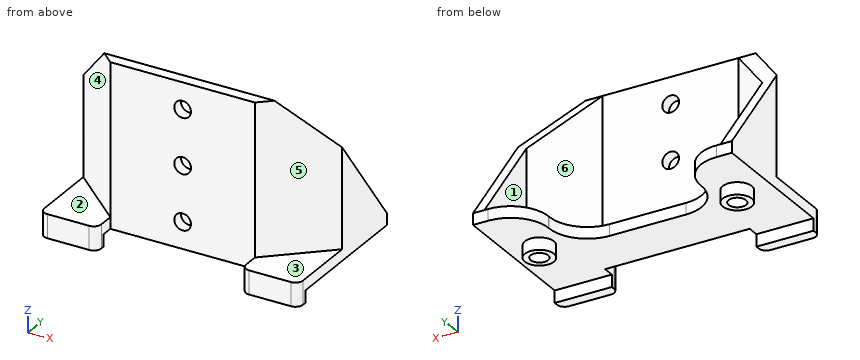
from build123d import *

# Parameters (mm, degrees)
F4_DEPTH       = 21.4
F5_DEPTH       = 1.5
F1_R           = 1.9
F6_DEPTH       = 1.6
F8_DEPTH       = 17.001
F8_DEPTH_BACK  = 17.001
F9_R           = 1.15
F10_DEPTH      = 21.401
F10_DEPTH_BACK = 1.601
F11_R          = 1.1
F12_DEPTH      = 1.5
F15_DEPTH      = 1.5
F14_W          = 7.5
F14_H          = 1.5
F16_DEPTH      = 1.6
F17_R          = 1
F18_R          = 5


with BuildPart() as f4:
    # F3 (on face) → F4 (new body)
    with BuildSketch(Plane.XY):
        Polygon((-15.5, 10), (-17, 10), (-17, 0), (-9.5, -6.7), (0, -6.7), (9.5, -6.7), (17, 0), (17, 10), (15.5, 10), (15.5, 0.6713676939), (8.927573477, -5.2), (0, -5.2), (-8.927573477, -5.2), (-15.5, 0.6713676939), align=None)
    extrude(amount=F4_DEPTH)

    # F2 (on Top) → F5 (join)
    with BuildSketch(Plane.XY):
        Polygon((-17, 0), (-9.5, -6.7), (0, -6.7), (9.5, -6.7), (17, 0), (17, 10), (10, 10), (10, -0.1), (0, -0.1), (-10, -0.1), (-10, 10), (-17, 10), align=None)
    extrude(amount=F5_DEPTH)

    # F1 (on Top) → F6 (join)
    with BuildSketch(Plane.XY):
        with Locations((-13, 2)):
            Circle(F1_R)
        with Locations((13, 2)):
            Circle(F1_R)
    extrude(amount=-F6_DEPTH)

    # F7 (on Right) → F8 (cut, two sides)
    with BuildSketch(Plane.YZ) as f8_sk:
        Polygon((-5.2, 21.4), (10, 1.5), (10, 21.4), align=None)
    extrude(amount=-F8_DEPTH, mode=Mode.SUBTRACT)
    extrude(f8_sk.sketch, amount=F8_DEPTH_BACK, mode=Mode.SUBTRACT)

    # F9 (on Top) → F10 (cut, two sides)
    with BuildSketch(Plane.XY) as f10_sk:
        with Locations((13, 2)):
            Circle(F9_R)
        with Locations((-13, 2)):
            Circle(F9_R)
    extrude(amount=F10_DEPTH, mode=Mode.SUBTRACT)
    extrude(f10_sk.sketch, amount=-F10_DEPTH_BACK, mode=Mode.SUBTRACT)

    # F11 (on face) → F12 (cut, through all)
    with BuildSketch(Plane.XZ.offset(6.7)):
        with Locations((0, 3.475)):
            Circle(F11_R)
        with Locations((0, 17.925)):
            Circle(F11_R)
        with Locations((0, 10.7)):
            Circle(F11_R)
    extrude(amount=-F12_DEPTH, mode=Mode.SUBTRACT)

    # F13 (on Top) → F15 (join)
    with BuildSketch(Plane.XY):
        Polygon((-17, 0), (-17, -9.7), (-9.5, -9.7), (-9.5, -6.7), align=None)
        Polygon((9.5, -9.7), (17, -9.7), (17, 0), (9.5, -6.7), align=None)
    extrude(amount=F15_DEPTH)

    # F14 (on face) → F16 (join)
    with BuildSketch(Plane.XY):
        with Locations((-13.25, -8.95)):
            Rectangle(F14_W, F14_H)
        with Locations((13.25, -8.95)):
            Rectangle(F14_W, F14_H)
    extrude(amount=-F16_DEPTH)

    # F17
    f17_edges = [f4.edges().sort_by_distance(p)[0] for p in [
        (17, -9.7, -0.05),
        (-17, -9.7, -0.05),
        (-9.5, -9.7, -0.05),
        (9.5, -9.7, -0.05),
    ]]
    fillet(f17_edges, radius=F17_R)

    # F18
    f18_edges = [f4.edges().sort_by_distance(p)[0] for p in [
        (10, -0.1, 0.75),
        (10, 10, 0.75),
        (-10, -0.1, 0.75),
        (-10, 10, 0.75),
    ]]
    fillet(f18_edges, radius=F18_R)


solid = f4.part
The model under review builds one solid part; all positions refer to its coordinate system, in mm. Face numbers are marked on the shaded views. A direction names the side the tool comes from. Round coordinates to 2 decimals unless told otherwise and drop trailing zeros. Write each loop counter-clockwise with the first axis right and the second up, starting at its lowest first coordinate (ties: lowest second). Pieces come first, ordered by that corner, then holes. Notation, with made-up numbers: M -16,50.25 L -8,50.25 A21 cw -8,89.25 Z; hole C -25.75,6 d5. An arc over 180 degrees is marked long. Answer as CSV lines item,"result". Start each with the question number.
Q1. Clearance check with flat-ended pins moving along their axes: P1, Ø3, axis at x = 13, y = 2, coming from the +Z side; P2, Ø12, axis at x = 7.5, z = 9, coming from the +Y side; P3, Ø3.5, axis at x = 0, z = 10.7, coming from the +Y side; P4, Ø8, axis at x = 14.5, y = -5.5, coming from the +Z side. State where each tip first meets the part, or that it passes through.
Q2. Consider section C-C, the plane z = 10.7. Give the boundary of the cut face in (x, y), then the cut area to 3 significant figures.
Q3. Consider section A-A, the plane x = 0. Give the boundary of the cut face in (y, z) (3 decimals), then the cut area to 4 significant figures.
Q4. Consider section D-D, the plane y = 2. Give the boundary of the cut face in (x, z).
Q5. Consider section B-B, the plane y = 9. Give the boundary of the cut face in (x, z).
Q6. Tool access review of the marked faces 1, 2 and 3: name each direction out of +Z, -Z, +X, -X, +Y, -Y from which nothing blocks a thin tool from reaching the whole face with its end or side.
Q7. The part is to be moulded in two halves that separate along X. For the marked faces 4, 5 and 6, say which applies: +X half, -X half, draft (parallel to the pull), parting line (faces both ways), or undercut.
Q8. Wall thickness on line 1 along Y through (x, z) = (13, -0.7); line 2 along Z through (x, y) = (0, -5.75) (3 decimals); line 3 along X through (y, z) = (2, 0.55): over which ranges is each line inside the solid? List them lowest first.
Result set:
1,P1,"stops at z = 1.5"
1,P2,"stops at y = -1.12"
1,P3,"stops at y = -5.2"
1,P4,"stops at z = 21.4"
2,outline,"M -17,0 L -9.5,-6.7 L -1.1,-6.7 L -1.1,-5.2 L -8.93,-5.2 L -15.5,0.67 L -15.5,2.97 L -17,2.97 Z; M 1.1,-6.7 L 9.5,-6.7 L 17,0 L 17,2.97 L 15.5,2.97 L 15.5,0.67 L 8.93,-5.2 L 1.1,-5.2 Z"
2,area,"60.6 mm²"
3,outline,"M -6.7,0 L -0.1,0 L -0.1,1.5 L -5.2,1.5 L -5.2,2.375 L -6.7,2.375 Z; M -6.7,4.575 L -5.2,4.575 L -5.2,9.6 L -6.7,9.6 Z; M -6.7,11.8 L -5.2,11.8 L -5.2,16.825 L -6.7,16.825 Z; M -6.7,19.025 L -5.2,19.025 L -5.2,21.4 L -6.7,21.4 Z"
3,area,"29.85 mm²"
4,outline,"M -17,0 L -14.9,0 L -14.9,-1.6 L -14.15,-1.6 L -14.15,1.5 L -15.5,1.5 L -15.5,11.97 L -17,11.97 Z; M -11.85,-1.6 L -11.1,-1.6 L -11.1,0 L -9.07,0 L -9.07,1.5 L -11.85,1.5 Z; M 9.07,0 L 11.1,0 L 11.1,-1.6 L 11.85,-1.6 L 11.85,1.5 L 9.07,1.5 Z; M 14.15,-1.6 L 14.9,-1.6 L 14.9,0 L 17,0 L 17,11.97 L 15.5,11.97 L 15.5,1.5 L 14.15,1.5 Z"
5,outline,"M -17,0 L -12,0 L -12,1.5 L -15.5,1.5 L -15.5,2.81 L -17,2.81 Z; M 12,0 L 17,0 L 17,2.81 L 15.5,2.81 L 15.5,1.5 L 12,1.5 Z"
6,face 1,"+Z, +Y"
6,face 2,"+Z, -X, -Y"
6,face 3,"+Z, +X, -Y"
7,face 4,"-X half"
7,face 5,"+X half"
7,face 6,"undercut"
8,line 1,"y = -9.7 to -8.2, 0.1 to 0.85, 3.15 to 3.9"
8,line 2,"z = 0 to 2.375, 4.575 to 9.6, 11.8 to 16.825, 19.025 to 21.4"
8,line 3,"x = -17 to -14.15, -11.85 to -9.07, 9.07 to 11.85, 14.15 to 17"
